Work out the finished part from the listing and answer in its coordinate system (mm). Round coordinates to 2 decimals unless told otherwise and drop trailing zeros. Loops run counter-clockwise (first coordinate to the right, second up) from the corner with the lowest first, then second, coordinate; pieces in that order, holes last. Notation, with made-up numbers: (36, 47.5) - (80, 47.5) arc R24 ccw to (80, 73.5) - close; hole circle Ø7 at (-15.75, 19.25). An arc over 180 degrees is marked (long way). Use CSV: the item, a comma, the result in double quotes. Start each with the question number.
from build123d import *


with BuildPart() as f1:
    # F0 (on Front) → F1 (revolve)
    with BuildSketch(Plane.XZ):
        with BuildLine():
            Line((-9.75, -1.675), (-9.75, 1.675))
            ThreePointArc((-9.75, 1.675), (-10.18934, 2.73566), (-11.25, 3.175))
            Line((-11.25, 3.175), (-12.75, 3.175))
            Line((-12.75, 3.175), (-12.75, 2.175))
            Line((-12.75, 2.175), (-12.217371, 2.175))
            ThreePointArc((-12.217371, 2.175), (-11.289957, 1.258655), (-10.95, 0))
            ThreePointArc((-10.95, 0), (-11.289957, -1.258655), (-12.217371, -2.175))
            Line((-12.217371, -2.175), (-12.75, -2.175))
            Line((-12.75, -2.175), (-12.75, -3.175))
            Line((-12.75, -3.175), (-11.25, -3.175))
            ThreePointArc((-11.25, -3.175), (-10.18934, -2.73566), (-9.75, -1.675))
        make_face()
    revolve(axis=Axis((0, 0, 0.475), (0, 0, -1)))


solid = f1.part
Item 1: A cutting plane is placed at D-D (z = 2.75). Determine the outline of the cut face in (x, y).
Item 2: Each of these flat-tipped pins is pushed along its axis until it touches: pin 1 Ø2 at (x, z) = (7.5, 0.5) entering from +Y; pin 2 Ø13 at (x, y) = (-1, -5) entering from +Z (3 decimals); pin 3 Ø1.5 at (x, y) = (6.5, 7) entering from -Z; pin 4 Ø1.5 at (x, y) = (-9, 2.5) entering from +Z. Where does it stop, or does it pass through?
Item 3: Find the intervals of material crossed by probe 1 along Y at (x, z) = (7.5, 2.75); probe 2 along Y at (x, z) = (3, 1.5); probe 3 along X at (y, z) = (6, 0), in increasing order. Write a range as [from, to].
Item 4: A cutting plane is placed at C-C (z = -0.5). Determine the outline of the cut face in (x, y).
Item 5: The mould has two halves that part along Y. Classify faces 1 (the cylindrical face through (2.764, -12.447, -2.682)), 2 (the flat face through (7, -9, 3.175)), 3 (the cylindrical face through (1.269, 9.667, 0.023)): pulls with the +Y half, pulls with the -Y half, needs draft (parallel to the pull), parting line crosses it, or undercut.
Item 6: A cutting plane is placed at A-A (x = 0). Determine the outline of the cut face in (y, z) (3 decimals), plus the area to 3 significant figures.
Result sheet:
1,outline,"circle Ø25.5 at (0, 0); hole circle Ø20.41 at (0, 0)"
2,pin 1,"y = 8.98"
2,pin 2,"z = 3.175"
2,pin 3,"z = -2.84"
2,pin 4,"z = 2.63"
3,probe 1,"[-10.31, -6.92], [6.92, 10.31]"
3,probe 2,"[-11.05, -9.28], [9.28, 11.05]"
3,probe 3,"[-9.16, -7.69], [7.69, 9.16]"
4,outline,"circle Ø22 at (0, 0); hole circle Ø19.5 at (0, 0)"
5,face 1,"parting line crosses it"
5,face 2,"needs draft"
5,face 3,"undercut"
6,outline,"(-12.75, -3.175) - (-11.25, -3.175) arc R1.5 ccw to (-9.75, -1.675) - (-9.75, 1.675) arc R1.5 ccw to (-11.25, 3.175) - (-12.75, 3.175) - (-12.75, 2.175) - (-12.217, 2.175) arc R2.5 cw to (-10.95, 0) arc R2.5 cw to (-12.217, -2.175) - (-12.75, -2.175) - close; (9.75, -1.675) arc R1.5 ccw to (11.25, -3.175) - (12.75, -3.175) - (12.75, -2.175) - (12.217, -2.175) arc R2.5 cw to (10.95, 0) arc R2.5 cw to (12.217, 2.175) - (12.75, 2.175) - (12.75, 3.175) - (11.25, 3.175) arc R1.5 ccw to (9.75, 1.675) - close"
6,area,"23.7 mm^2"
